from build123d import *

# Parameters (mm, degrees)
SKETCH_1_W      = 2
SKETCH_1_H      = 5
SKETCH_1_W_2    = 41.7
SKETCH_1_H_2    = 25
EXTRUDE_1_DEPTH = 15
EXTRUDE_2_DEPTH = 41.7
SKETCH_4_W      = 5
SKETCH_4_H      = 25.88190451
EXTRUDE_4_DEPTH = 18
EXTRUDE_3_REACH = 58.078
SKETCH_3_W      = 2
SKETCH_3_H      = 5


with BuildPart() as part:
    # 草圖1 → 填料-伸長1 (new body)
    with BuildSketch(Plane(origin=(0, 0, 0), x_dir=(1, 0, 0), z_dir=(0, 1, 0))):
        with Locations((-1, 12.5)):
            Rectangle(SKETCH_1_W, SKETCH_1_H)
        with Locations((20.85, 12.5)):
            Rectangle(SKETCH_1_W_2, SKETCH_1_H_2)
        with Locations((42.7, 12.5)):
            Rectangle(SKETCH_1_W, SKETCH_1_H)
    extrude(amount=EXTRUDE_1_DEPTH)

    # 草圖2 → 填料-伸長2 (add)
    with BuildSketch(Plane(origin=(41.7, 0, 0), x_dir=(0, 0, -1), z_dir=(1, 0, 0))):
        Polygon((0, 15), (25, 21.698729811), (25, 15), align=None)
    extrude(amount=-EXTRUDE_2_DEPTH)

    # 草圖4 → 填料-伸長4 (add, along a direction that is not the sketch's normal)
    with BuildSketch(Plane(origin=(0, 13.995190528, 3.75), x_dir=(1, 0, 0), z_dir=(0, 0.9659258262890681, 0.25881904510252157))):
        with Locations((2.5, 16.823237932)):
            Rectangle(SKETCH_4_W, SKETCH_4_H)
        with Locations((39.2, 16.823237932)):
            Rectangle(SKETCH_4_W, SKETCH_4_H)
    extrude(amount=EXTRUDE_4_DEPTH, dir=(0, 1, 0))

    # 填料-伸長3: up to this plane
    extrude_3_end = Plane(origin=(0, 31.995190528, 3.75), z_dir=(0, 0.9659258262890682, 0.2588190451025215))
    # 草圖3 → 填料-伸長3 (add, up to the surface)
    with BuildSketch(Plane(origin=(0, 15, 0), x_dir=(1, 0, 0), z_dir=(0, 1, 0)), mode=Mode.PRIVATE) as extrude_3_sk1:
        with Locations((42.7, 12.5)):
            Rectangle(SKETCH_3_W, SKETCH_3_H)
    extrude_3_tool1 = split(extrude(extrude_3_sk1.sketch, amount=EXTRUDE_3_REACH, mode=Mode.PRIVATE), bisect_by=extrude_3_end, keep=Keep.BOTH, mode=Mode.PRIVATE)
    add(extrude_3_tool1.solids().sort_by_distance((42.7, 15, -12.5))[0])
    # 草圖3 → 填料-伸長3 (add, up to the surface)
    with BuildSketch(Plane(origin=(0, 15, 0), x_dir=(1, 0, 0), z_dir=(0, 1, 0)), mode=Mode.PRIVATE) as extrude_3_sk2:
        with Locations((-1, 12.5)):
            Rectangle(SKETCH_3_W, SKETCH_3_H)
    extrude_3_tool2 = split(extrude(extrude_3_sk2.sketch, amount=EXTRUDE_3_REACH, mode=Mode.PRIVATE), bisect_by=extrude_3_end, keep=Keep.BOTH, mode=Mode.PRIVATE)
    add(extrude_3_tool2.solids().sort_by_distance((-1, 15, -12.5))[0])


solid = part.part
CAD build for the part. Positions are in the model's coordinates, mm. A direction names the side the tool comes from. Round coordinates to 2 decimals unless told otherwise and drop trailing zeros. Loops run counter-clockwise (first coordinate to the right, second up) from the corner with the lowest first, then second, coordinate; pieces in that order, holes last. Notation, with made-up numbers: M -10,-13.5 L -2,-13.5 A10 ccw -2,-9.5 Z; hole C 15.25,-36 d10. An arc over 180 degrees is marked long. One line per question, with ' | ' between items. Start each with the question number.
Item 1: Cut at D-D, the plane x = 15. Write the cut outline in (y, z).
Item 2: Cut at A-A, the plane y = 30. Write the cut outline in (x, z), plus the area to 3 significant figures.
Item 3: Cut at B-B, the plane z = -4.5. Write the cut outline in (x, y).
Item 4: Pin check, flat tips, straight feed: pin 1 Ø6 at (x, z) = (9.5, -20) entering from +Y; pin 2 Ø4 at (y, z) = (8, -22) entering from -X; pin 3 Ø2 at (x, z) = (21.5, -19) entering from +Y. Stop position of each tip, or through.
Item 5: Two-plate mould, pull along X, no slides. Class faces 5 (the flat face through (2.327, 36.396, -12.675)), 6 (the flat face through (0, 16, -5)), 7 (the flat face through (41.7, 18, -5)), 8 (the flat face through (5, 27, -12)): pulls with the +X half, pulls with the -X half, needs draft (parallel to the pull), parting line crosses it, or undercut.
Item 6: Cut at C-C, the plane y = 7.5. Write the cut outline in (x, z), plus the area to 3 significant figures.
Item 7: Wall check: line 1 (X direction, y = 26, z = -18.75); line 2 (X direction, y = 34, z = -10.25); line 3 (Z direction, x = 42, y = 9.5). Give the ranges that are in metal, low to high.
Item 8: Which spindle directions (+Z, -Z, +X, -X, +Y, -Y) get a long thin tool onto all of the face, cutting with end or side? Do faces 1 (the flat face through (41.7, 20, -20)), 2 (the flat face through (0, 18, -20)), 3 (the flat face through (36.7, 27, -12)), 4 (the flat face through (-1, 18, -10)). Say none if no direction does.
Responses:
1) outline: M 0,-25 L 21.7,-25 L 15,0 L 0,0 Z
2) outline: M -2,-15 L 0,-15 L 0,-25 L 5,-25 L 5,0 L 0,0 L 0,-10 L -2,-10 Z; M 36.7,-25 L 41.7,-25 L 41.7,-15 L 43.7,-15 L 43.7,-10 L 41.7,-10 L 41.7,0 L 36.7,0 Z | area: 270 mm²
3) outline: M 0,0 L 41.7,0 L 41.7,34.21 L 36.7,34.21 L 36.7,16.21 L 5,16.21 L 5,34.21 L 0,34.21 Z
4) pin 1: stops at y = 21.16 | pin 2: stops at x = 0 | pin 3: stops at y = 20.36
5) face 5: needs draft | face 6: pulls with the -X half | face 7: pulls with the +X half | face 8: undercut
6) outline: M -2,-15 L 0,-15 L 0,-25 L 41.7,-25 L 41.7,-15 L 43.7,-15 L 43.7,-10 L 41.7,-10 L 41.7,0 L 0,0 L 0,-10 L -2,-10 Z | area: 1,060 mm²
7) line 1: x = 0 to 5, 36.7 to 41.7 | line 2: x = -2 to 5, 36.7 to 43.7 | line 3: z = -15 to -10
8) face 1: -Z, +X, +Y, -Y | face 2: -Z, -X, +Y, -Y | face 3: +Z, +Y | face 4: +Z, -X, +Y, -Y
